```python
from build123d import *

# Parameters (mm, degrees)
SKETCH2_W           = 35
SKETCH2_H           = 35
BOSS_EXTRUDE1_DEPTH = 15
SKETCH3_W           = 35
SKETCH3_H           = 12
BOSS_EXTRUDE2_DEPTH = 35
SKETCH4_R           = 9
CUT_EXTRUDE1_DEPTH  = 2
SKETCH5_R           = 3
CUT_EXTRUDE2_DEPTH  = 14
SKETCH6_R           = 1.5
CUT_EXTRUDE3_DEPTH  = 58.751623354
SKETCH8_R           = 1.7
CUT_EXTRUDE4_DEPTH  = 43.866070499


with BuildPart() as part:
    # Sketch2 → Boss-Extrude1 (new body)
    with BuildSketch(Plane.XY):
        Rectangle(SKETCH2_W, SKETCH2_H)
    extrude(amount=BOSS_EXTRUDE1_DEPTH)

    # Sketch3 → Boss-Extrude2 (add)
    with BuildSketch(Plane.XY.offset(15)):
        with Locations((0, -11.5)):
            Rectangle(SKETCH3_W, SKETCH3_H)
    extrude(amount=BOSS_EXTRUDE2_DEPTH)

    # Sketch4 → Cut-Extrude1 (cut)
    with BuildSketch(Plane(origin=(0, -5.5, 0), x_dir=(1, 0, 0), z_dir=(0, 1, 0))):
        with Locations(Location((0, -32.5, 0), (0, 0, 270))):
            Circle(SKETCH4_R)
    extrude(amount=-CUT_EXTRUDE1_DEPTH, mode=Mode.SUBTRACT)

    # Sketch5 → Cut-Extrude2 (cut)
    with BuildSketch(Plane(origin=(0, -7.5, 0), x_dir=(1, 0, 0), z_dir=(0, 1, 0))):
        with Locations(Location((0, -32.5, 0), (0, 0, 270))):
            Circle(SKETCH5_R)
    extrude(amount=-CUT_EXTRUDE2_DEPTH, mode=Mode.SUBTRACT)

    # Sketch6 → Cut-Extrude3 (cut, through all)
    with BuildSketch(Plane(origin=(0, -5.5, 0), x_dir=(1, 0, 0), z_dir=(0, 1, 0))):
        with Locations(Location((0, -21.5, 0), (0, 0, 270))):
            Circle(SKETCH6_R)
        with Locations(Location((0, -43.5, 0), (0, 0, 90))):
            Circle(SKETCH6_R)
        with Locations(Location((-11, -32.5, 0), (0, 0, 270))):
            Circle(SKETCH6_R)
        with Locations(Location((11, -32.5, 0), (0, 0, 270))):
            Circle(SKETCH6_R)
    extrude(amount=-CUT_EXTRUDE3_DEPTH, mode=Mode.SUBTRACT)

    # Sketch8 → Cut-Extrude4 (cut, through all)
    with BuildSketch(Plane.XY.offset(15)):
        with Locations((-8.75, 0.5)):
            Circle(SKETCH8_R)
        with Locations((8.75, 0.5)):
            Circle(SKETCH8_R)
        with Locations((8.75, 11.5)):
            Circle(SKETCH8_R)
        with Locations((-8.75, 11.5)):
            Circle(SKETCH8_R)
    extrude(amount=-CUT_EXTRUDE4_DEPTH, mode=Mode.SUBTRACT)


solid = part.part
```
Could you check a few things on this model? Use its own coordinates, in mm. A direction names the side the tool comes from. Give positions to 0.01 mm unless a question says otherwise; leave off trailing zeros. Order: outer loops, then holes, each group sorted by start corner. A loop starts at its lowest first (then second) coordinate and runs counter-clockwise, first axis right, second up.
Q1. Suppose I cut it at A-A, the plane z = 43.5. Write out the boundary of the cut face in (x, y).
Q2. For faces 5 (the flat face through (0, 0, 0)), 6 (the flat face through (2, -7.5, 30)), 7 (the flat face through (0, 6, 15)), which set-ups out of +Z, -Z, +X, -X, +Y, -Y let a thin tool reach every point of the face, with its end or its side?
Q3. Suppose I cut it at D-D, the plane z = 32.5. Write out the boundary of the cut face in (x, y), and give its area (3 significant figures).
Q4. I'm going to push flat-ended pins straight in: P1, Ø1.5, axis at x = 6.5, y = -9.5, coming from the -Z side; P2, Ø10, axis at x = -5, y = 11.5, coming from the +Z side; P3, Ø12, axis at x = -10, z = 30.5, coming from the +Y side; P4, Ø5.5, axis at x = 3.5, z = 30.5, coming from the +Y side. Where does each tip first touch, or does it pass through?
Q5. Suppose I cut it at C-C, the plane y = 0.5. Write out the boundary of the cut face in (x, z), and give its area (3 significant figures).
Q6. We'd pull the mould along Y, two halves only. Please class faces 1 (the cylindrical face through (-10.1, -0.53, 7.6)), 2 (the cylindrical face through (11, -11, 31)), 3 (the flat face through (-4, -5.5, 24)), 4 (the flat face through (0, -17.5, 25)): +Y half, -Y half, draft (parallel to the pull), parting line (faces both ways), or undercut.
Q7. Suppose I cut it at B-B, the plane x = 0. Write out the boundary of the cut face in (y, z), and give its area (3 significant figures).
Q8. If I drill on line 1 along Y through (x, z) = (8.75, 6); line 2 along X through (y, z) = (-14.5, 32.5); line 3 along X through (y, z) = (-7, 32.5), over which ranges is the centre line in solid material (lowest first)?
Solution:
1. outline: (-17.5, -17.5) - (-1.5, -17.5) - (-1.5, -5.5) - (-17.5, -5.5) - close; (1.5, -17.5) - (17.5, -17.5) - (17.5, -5.5) - (1.5, -5.5) - close
2. face 5: -Z, +X, -X, +Y, -Y
2. face 6: +Y
2. face 7: +Z, +X, -X, +Y
3. outline: (-17.5, -17.5) - (-12.5, -17.5) - (-12.5, -5.5) - (-17.5, -5.5) - close; (-9.5, -17.5) - (-3, -17.5) - (-3, -7.5) - (-9, -7.5) - (-9, -5.5) - (-9.5, -5.5) - close; (3, -17.5) - (9.5, -17.5) - (9.5, -5.5) - (9, -5.5) - (9, -7.5) - (3, -7.5) - close; (12.5, -17.5) - (17.5, -17.5) - (17.5, -5.5) - (12.5, -5.5) - close
3. area: 252 mm2
4. P1: stops at z = 0
4. P2: stops at z = 15
4. P3: stops at y = -5.5
4. P4: stops at y = -7.5
5. outline: (-17.5, 0) - (-10.45, 0) - (-10.45, 15) - (-17.5, 15) - close; (-7.05, 0) - (7.05, 0) - (7.05, 15) - (-7.05, 15) - close; (10.45, 0) - (17.5, 0) - (17.5, 15) - (10.45, 15) - close
5. area: 423 mm2
6. face 1: undercut
6. face 2: draft
6. face 3: +Y half
6. face 4: -Y half
7. outline: (-17.5, 0) - (17.5, 0) - (17.5, 15) - (-5.5, 15) - (-5.5, 20) - (-17.5, 20) - close; (-17.5, 23) - (-5.5, 23) - (-5.5, 23.5) - (-7.5, 23.5) - (-7.5, 29.5) - (-17.5, 29.5) - close; (-17.5, 35.5) - (-7.5, 35.5) - (-7.5, 41.5) - (-5.5, 41.5) - (-5.5, 42) - (-17.5, 42) - close; (-17.5, 45) - (-5.5, 45) - (-5.5, 50) - (-17.5, 50) - close
7. area: 777 mm2
8. line 1: y = -17.5 to -1.2, 2.2 to 9.8, 13.2 to 17.5
8. line 2: x = -17.5 to -12.5, -9.5 to -3, 3 to 9.5, 12.5 to 17.5
8. line 3: x = -17.5 to -12.5, -9.5 to -9, 9 to 9.5, 12.5 to 17.5
